Build history of the part. All positions in model axes, mm. Face numbers are marked on the shaded views. A direction names the side the tool comes from. Coordinates: 2 decimals unless noted, no trailing zeros. Order: outer loops, then holes, each group sorted by start corner. A loop starts at its lowest first (then second) coordinate and runs counter-clockwise, first axis right, second up. Notation, with made-up numbers: M 89.25,60 L 95.25,60 A31 ccw 95.25,85 Z; hole C 38.5,-4.5 d5. An arc over 180 degrees is marked long. Use a Markdown table: item, result. Add a question column.
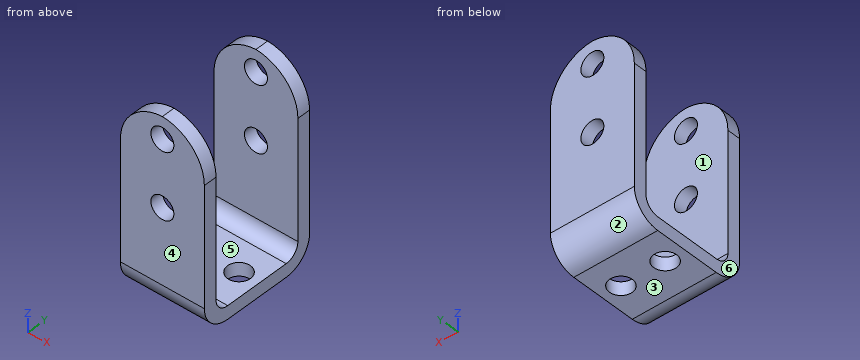
from build123d import *

# Parameters (mm, degrees)
SKETCH1_W                      = 19
SKETCH1_H                      = 27
BASE_FLANGE1_DEPTH             = 3
EDGE_FLANGE1_STRIP_W           = 18
EDGE_FLANGE1_STRIP_H           = 3
EDGE_FLANGE1_STRIP_CUT_DEPTH   = 19
EDGE_FLANGE1_STRIP_2_W         = 18
EDGE_FLANGE1_STRIP_2_H         = 3
EDGE_FLANGE1_STRIP_CUT_2_DEPTH = 19
EDGE_FLANGE1_DEPTH             = 19
EDGE_FLANGE1_BEND_DEPTH        = 19
SKETCH12_R                     = 2.6
CUT_EXTRUDE1_DEPTH             = 10
SKETCH13_R                     = 2.6
CUT_EXTRUDE2_DEPTH             = 50.185871955
FILLET1_R                      = 10


# Sheet-metal steps are written as plain solids
with BuildPart() as part:
    # Sketch1 → Base-Flange1 (new body)
    with BuildSketch(Plane.XY):
        Rectangle(SKETCH1_W, SKETCH1_H)
    extrude(amount=-BASE_FLANGE1_DEPTH)

    # Edge-Flange1 strip (across the edge) → Edge-Flange1 strip cut (cut)
    with BuildSketch(Plane(origin=(9.5, 13.5, 0), x_dir=(0, -1, 0), z_dir=(-1, 0, 0))):
        with Locations((-3, -1.5)):
            Rectangle(EDGE_FLANGE1_STRIP_W, EDGE_FLANGE1_STRIP_H)
    extrude(amount=EDGE_FLANGE1_STRIP_CUT_DEPTH, mode=Mode.SUBTRACT)

    # Edge-Flange1 strip 2 (across the edge) → Edge-Flange1 strip cut 2 (cut)
    with BuildSketch(Plane(origin=(-9.5, -13.5, 0), x_dir=(0, 1, 0), z_dir=(1, 0, 0))):
        with Locations((-3, -1.5)):
            Rectangle(EDGE_FLANGE1_STRIP_2_W, EDGE_FLANGE1_STRIP_2_H)
    extrude(amount=EDGE_FLANGE1_STRIP_CUT_2_DEPTH, mode=Mode.SUBTRACT)

    # Edge-Flange1 section (across the edge) → Edge-Flange1 (add)
    with BuildSketch(Plane(origin=(9.5, 13.5, 0), x_dir=(0, -1, 0), z_dir=(-1, 0, 0))):
        with BuildLine():
            Line((0, 3), (0, 40))
            Line((0, 40), (3, 40))
            Line((3, 40), (3, 3))
            ThreePointArc((3, 3), (3.878679656, 0.878679656), (6, 0))
            Line((6, 0), (6, -3))
            ThreePointArc((6, -3), (1.757359313, -1.242640687), (0, 3))
        make_face()
    extrude(amount=EDGE_FLANGE1_DEPTH)

    # Edge-Flange1 section 2 (across the edge) → Edge-Flange1 bend (add)
    with BuildSketch(Plane(origin=(-9.5, -13.5, 0), x_dir=(0, 1, 0), z_dir=(1, 0, 0))):
        with BuildLine():
            Line((0, 3), (0, 40))
            Line((0, 40), (3, 40))
            Line((3, 40), (3, 3))
            ThreePointArc((3, 3), (3.878679656, 0.878679656), (6, 0))
            Line((6, 0), (6, -3))
            ThreePointArc((6, -3), (1.757359313, -1.242640687), (0, 3))
        make_face()
    extrude(amount=EDGE_FLANGE1_BEND_DEPTH)

    # Sketch12 → Cut-Extrude1 (cut)
    with BuildSketch(Plane.XY):
        with Locations((5, 0.5)):
            Circle(SKETCH12_R)
        with Locations((-5, 0.5)):
            Circle(SKETCH12_R)
    extrude(amount=-CUT_EXTRUDE1_DEPTH, mode=Mode.SUBTRACT)

    # Sketch13 → Cut-Extrude2 (cut, through all)
    with BuildSketch(Plane(origin=(0, 13.5, 0), x_dir=(1, 0, 0), z_dir=(0, 1, 0))):
        with Locations(Location((0, -35, 0), (0, 0, 270))):
            Circle(SKETCH13_R)
        with Locations(Location((0, -20, 0), (0, 0, 270))):
            Circle(SKETCH13_R)
    extrude(amount=-CUT_EXTRUDE2_DEPTH, mode=Mode.SUBTRACT)

    # Fillet1
    # the kernel refuses this fillet: 10 mm, written as the material it takes off along each edge
    with BuildSketch(Plane(origin=(-9.5, -38.5, 40), x_dir=(0, 0, -1), z_dir=(0, 1, 0)), Plane(origin=(9.5, -38.5, 40), x_dir=(-1, 0, 0), z_dir=(0, 1, 0))) as fillet1_piece_1:
        with BuildLine():
            CenterArc((FILLET1_R, -FILLET1_R), FILLET1_R, 90, 90)
            Line((0, -FILLET1_R), (0, 0))
            Line((0, 0), (FILLET1_R, 0))
        make_face()
    extrude(amount=53, mode=Mode.SUBTRACT)
    with BuildSketch(Plane(origin=(-9.5, 38.5, 40), x_dir=(0, 0, -1), z_dir=(0, -1, 0)), Plane(origin=(9.5, 38.5, 40), x_dir=(-1, 0, 0), z_dir=(0, -1, 0))) as fillet1_piece_2:
        with BuildLine():
            CenterArc((FILLET1_R, FILLET1_R), FILLET1_R, 180, 90)
            Line((0, FILLET1_R), (0, 0))
            Line((0, 0), (FILLET1_R, 0))
        make_face()
    extrude(amount=53, mode=Mode.SUBTRACT)


solid = part.part
(1) Slice it at D-D on x = 1.75. Give the cut face in (y, z).
(2) Which spindle directions (+Z, -Z, +X, -X, +Y, -Y) get a long thin tool onto all of the face, cutting with end or side? Do the marked faces 5 and 6. Say none if no direction does.
(3) Slice it at C-C on x = -6.5. Give the cut face in (y, z).
(4) Mould opens along Y. For the marked faces 1, 2, 3 and 4 say: released by +Y, released by -Y, zero draft, split by the parting line, or undercut.
(5) Drill centre lines: line 1 along Y through (x, z) = (7.75, 18.5); line 2 along X through (y, z) = (-11.9, 20); line 3 along Z through (x, y) = (4.75, 7). Where is each one in solid material? Low to high. Write a range as from..to.
(6) Slice it at B-B on z = 14. Give the cut face in (x, y).
(7) Drop a flat-ended pin along its axis: P1, Ø2, axis at x = -7.5, y = 7, coming from the +Z side. Give the stop position or say it passes through.
(8) Slice it at A-A on z = 20. Give the cut face in (x, y), and give its area (3 significant figures).
Solutions:
| question | item | result |
|---|---|---|
| 1 | outline | M -13.5,3 A6 ccw -7.5,-3 L 7.5,-3 A6 ccw 13.5,3 L 13.5,18.08 L 10.5,18.08 L 10.5,3 A3 cw 7.5,0 L -7.5,0 A3 cw -10.5,3 L -10.5,18.08 L -13.5,18.08 Z; M -13.5,21.92 L -10.5,21.92 L -10.5,33.08 L -13.5,33.08 Z; M -13.5,36.92 L -10.5,36.92 L -10.5,39.74 L -13.5,39.74 Z; M 10.5,21.92 L 13.5,21.92 L 13.5,33.08 L 10.5,33.08 Z; M 10.5,36.92 L 13.5,36.92 L 13.5,39.74 L 10.5,39.74 Z |
| 2 | face 5 | +Z, +X, -X |
| 2 | face 6 | +Z, -Z, -X, +Y, -Y |
| 3 | outline | M -13.5,3 A6 ccw -7.5,-3 L -1.62,-3 L -1.62,0 L -7.5,0 A3 cw -10.5,3 L -10.5,37.14 L -13.5,37.14 Z; M 2.62,-3 L 7.5,-3 A6 ccw 13.5,3 L 13.5,37.14 L 10.5,37.14 L 10.5,3 A3 cw 7.5,0 L 2.62,0 Z |
| 4 | face 1 | undercut |
| 4 | face 2 | released by +Y |
| 4 | face 3 | zero draft |
| 4 | face 4 | released by -Y |
| 5 | line 1 | -13.5..-10.5, 10.5..13.5 |
| 5 | line 2 | -9.5..-2.6, 2.6..9.5 |
| 5 | line 3 | -3..0 |
| 6 | outline | M -9.5,-13.5 L 9.5,-13.5 L 9.5,-10.5 L -9.5,-10.5 Z; M -9.5,10.5 L 9.5,10.5 L 9.5,13.5 L -9.5,13.5 Z |
| 7 | P1 | z = 0.04 |
| 8 | outline | M -9.5,-13.5 L -2.6,-13.5 L -2.6,-10.5 L -9.5,-10.5 Z; M -9.5,10.5 L -2.6,10.5 L -2.6,13.5 L -9.5,13.5 Z; M 2.6,-13.5 L 9.5,-13.5 L 9.5,-10.5 L 2.6,-10.5 Z; M 2.6,10.5 L 9.5,10.5 L 9.5,13.5 L 2.6,13.5 Z |
| 8 | area | 82.8 mm² |
